Part model, mm, in its own coordinate system. Face numbers are marked on the shaded views. A direction names the side the tool comes from. Round coordinates to 2 decimals unless told otherwise and drop trailing zeros. Write each loop counter-clockwise with the first axis right and the second up, starting at its lowest first coordinate (ties: lowest second). Pieces come first, ordered by that corner, then holes. Notation, with made-up numbers: (17, 69) -> (23, 69) arc R17 ccw to (23, 87) -> close; hole circle Ø4 at (15, 79). An arc over 180 degrees is marked (long way). Return JSON: item names as keys, results as strings. Group by question number.
(1) Drill centre lines: L1, parallel to Z at x = 2.5, y = 8.5; L2, parallel to Z at x = -1.75, y = 9; L3, parallel to Y at x = -0.25, z = -3. Where is each one in solid material? Low to high. Write a range as from..to.
(2) Saw through at C-C (y = 8.25). List the corners of the cut face in (x, z), plus the area to 3 significant figures.
(3) Drop flat-ended pins along their axis: pin 1 Ø5 at (x, z) = (-4, -2) entering from +Y; pin 2 Ø1.5 at (x, y) = (5, 2.5) entering from +Z; pin 3 Ø5 at (y, z) = (1.5, 14.5) entering from +X; pin 4 Ø2 at (y, z) = (-1.5, -2) entering from -X. Give the stop position or say it passes through.
(4) Saw through at A-A (y = 0). List the corners of the cut face in (x, z).
(5) Saw through at D-D (x = -6.75). List the corners of the cut face in (y, z), plus the area to 3 significant figures.
(6) Tool access for the marked faces 1, 2 and 3: list every direction of +Z, -Z, +X, -X, +Y, -Y with a clear straight run to the whole face (end or side of a thin tool).
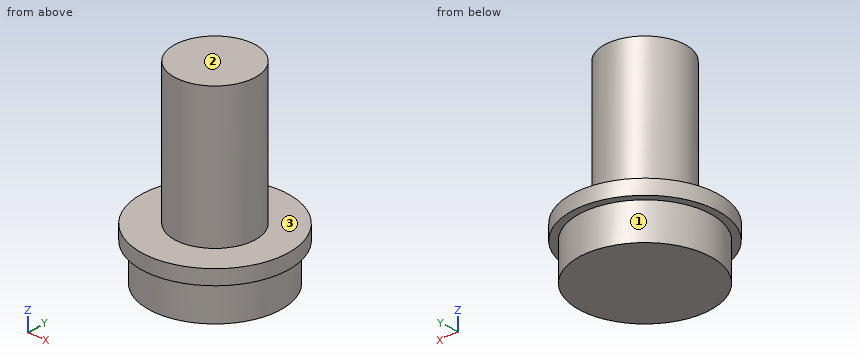
Autodesk Inventor part; units mm, degrees
ref_plane "YZ Plane" through (0, 0, 0) normal (1, 0, 0) x (0, 1, 0)
ref_plane "XZ Plane" through (0, 0, 0) normal (0, 1, 0) x (-1, 0, 0)
ref_plane "XY Plane" through (0, 0, 0) normal (0, 0, 1) x (1, 0, 0)
sketch "Эскиз1" plane through (0, 0, 0) normal (0, 0, 1) x (1, 0, 0)
  circle A0 centre (0, 0) radius 8.95
  circle A1 centre (0, 0) radius 9.95
  circle A2 centre (0, 0) radius 5.5
  dimension "d0" = 17.9
  dimension "d1" = 19.9
  dimension "d2" = 11
extrude "Выдавливание1" add sketch "Эскиз1" along normal blind 19 contours A2
extrude "Выдавливание2" add sketch "Эскиз1" against normal blind 2 contours A0 | A1 | A2
extrude "Выдавливание3" add sketch "Эскиз1" against normal blind 7 contours A0 | A2
properties part number "деталь ек"
Computed values:
{
 "1": {"L1": "-7..0", "L2": "-2..0", "L3": "-8.95..8.95"},
 "2": {"outline": "(-5.56, -2) -> (-3.47, -2) -> (-3.47, -7) -> (3.47, -7) -> (3.47, -2) -> (5.56, -2) -> (5.56, 0) -> (-5.56, 0) -> close", "area": "56.9 mm2"},
 "3": {"pin 1": "y = 9.84", "pin 2": "z = 19", "pin 3": "x = 5.5", "pin 4": "x = -9.94"},
 "4": {"outline": "(-9.95, -2) -> (-8.95, -2) -> (-8.95, -7) -> (8.95, -7) -> (8.95, -2) -> (9.95, -2) -> (9.95, 0) -> (5.5, 0) -> (5.5, 19) -> (-5.5, 19) -> (-5.5, 0) -> (-9.95, 0) -> close"},
 "5": {"outline": "(-7.31, -2) -> (-5.88, -2) -> (-5.88, -7) -> (5.88, -7) -> (5.88, -2) -> (7.31, -2) -> (7.31, 0) -> (-7.31, 0) -> close", "area": "88.0 mm2"},
 "6": {"face 1": "-Z", "face 2": "+Z, +X, -X, +Y, -Y", "face 3": "+Z"}
}
